```python
from build123d import *

# Parameters (mm, degrees)
SKETCH1_R           = 135.7
SKETCH1_R_2         = 4
BOSS_EXTRUDE1_DEPTH = 10.6
SKETCH3_R           = 4.3
SKETCH5_R           = 4.3


with BuildPart() as part:
    # Sketch1 → Boss-Extrude1 (new body)
    with BuildSketch(Plane(origin=(0, 0, 0), x_dir=(1, 0, 0), z_dir=(0, 1, 0))):
        with Locations(Location((0, 0, 0), (0, 0, 270))):
            Circle(SKETCH1_R)
        with Locations(Location((0, 0, 0), (0, 0, 270))):
            Circle(SKETCH1_R_2, mode=Mode.SUBTRACT)
        with BuildLine():
            Line((-9.028288874, 4.3), (-128.4, 4.3))
            ThreePointArc((-128.4, 4.3), (-111.259999551, 64.235990691), (-67.923909236, 109.047661846))
            Line((-67.923909236, 109.047661846), (-8.238053673, 5.668727518))
            ThreePointArc((-8.238053673, 5.668727518), (-8.660254038, 5), (-9.028288874, 4.3))
        make_face(mode=Mode.SUBTRACT)
        with BuildLine():
            Line((-9.028288874, -4.3), (-128.4, -4.3))
            ThreePointArc((-128.4, -4.3), (-111.259999551, -64.235990691), (-67.923909236, -109.047661846))
            Line((-67.923909236, -109.047661846), (-8.238053673, -5.668727518))
            ThreePointArc((-8.238053673, -5.668727518), (-8.660254038, -5), (-9.028288874, -4.3))
        make_face(mode=Mode.SUBTRACT)
        with BuildLine():
            Line((-0.790235201, 9.968727518), (-60.476090764, 113.347661846))
            ThreePointArc((-60.476090764, 113.347661846), (0, 128.471981381), (60.476090764, 113.347661846))
            Line((60.476090764, 113.347661846), (0.790235201, 9.968727518))
            ThreePointArc((0.790235201, 9.968727518), (0, 10), (-0.790235201, 9.968727518))
        make_face(mode=Mode.SUBTRACT)
        with BuildLine():
            Line((8.238053673, 5.668727518), (67.923909236, 109.047661846))
            ThreePointArc((67.923909236, 109.047661846), (111.259999551, 64.235990691), (128.4, 4.3))
            Line((128.4, 4.3), (9.028288874, 4.3))
            ThreePointArc((9.028288874, 4.3), (8.660254038, 5), (8.238053673, 5.668727518))
        make_face(mode=Mode.SUBTRACT)
        with BuildLine():
            Line((9.028288874, -4.3), (128.4, -4.3))
            ThreePointArc((128.4, -4.3), (111.259999551, -64.235990691), (67.923909236, -109.047661846))
            Line((67.923909236, -109.047661846), (8.238053673, -5.668727518))
            ThreePointArc((8.238053673, -5.668727518), (8.660254038, -5), (9.028288874, -4.3))
        make_face(mode=Mode.SUBTRACT)
        with BuildLine():
            Line((0.790235201, -9.968727518), (60.476090764, -113.347661846))
            ThreePointArc((60.476090764, -113.347661846), (0, -128.471981381), (-60.476090764, -113.347661846))
            Line((-60.476090764, -113.347661846), (-0.790235201, -9.968727518))
            ThreePointArc((-0.790235201, -9.968727518), (0, -10), (0.790235201, -9.968727518))
        make_face(mode=Mode.SUBTRACT)
    extrude(amount=BOSS_EXTRUDE1_DEPTH)

    # Sketch3 → Cut-Revolve1 (revolve, cut)
    with BuildSketch(Plane.XY, mode=Mode.PRIVATE) as cut_revolve1_sk:
        with Locations((135.7, 5.3)):
            Circle(SKETCH3_R)
    revolve(cut_revolve1_sk.sketch.rotate(Axis((0, 0, 0), (0, 1, 0)), 90), axis=Axis((0, 0, 0), (0, 1, 0)), mode=Mode.SUBTRACT)

    # Sketch5 → Revolve1 (revolve)
    with BuildSketch(Plane(origin=(0, 0, 0), x_dir=(0, 0, -1), z_dir=(1, 0, 0))):
        with Locations((135.7, 5.3)):
            Circle(SKETCH5_R)
    revolve(axis=Axis((0, 0, 0), (0, 1, 0)))


solid = part.part
```
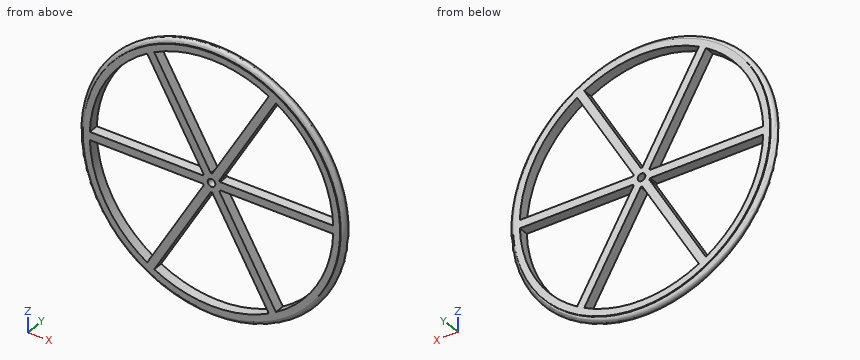
Could you check a few things on this model? Use its own coordinates, in mm. Give positions to 0.01 mm unless a question says otherwise; leave off trailing zeros. Order: outer loops, then holes, each group sorted by start corner. A loop starts at its lowest first (then second) coordinate and runs counter-clockwise, first axis right, second up.
Q1. I'm going to push flat-ended pins straight in: P1, Ø1, axis at x = 52.5, y = 4.5, coming from the +Z side; P2, Ø5.5, axis at x = -75, y = 6.5, coming from the +Z side; P3, Ø4, axis at x = -95, y = 9.5, coming from the -Z side. Where does each tip first touch, or does it pass through?
Q2. Suppose I cut it at C-C, the plane x = 122.5. Count the separate pieces of the cut face and the enclosed holes in it, and give its area (3 significant figures).
Q3. Suppose I cut it at B-B, the plane y = 3.5. Write out the boundary of the cut face in (x, z).
Q4. Suppose I cut it at A-A, the plane z = 0. Write out the boundary of the cut face in (x, y), and give its area (3 significant figures).
Q5. If I drill on line 1 along Z through (x, y) = (68, 6.75); line 2 along Z through (x, y) = (-45.5, 5); line 3 along Z through (x, y) = (21, 9.25), over which ranges is the centre line in solid material (lowest first)?
Solution:
1. P1: stops at z = 129.92
1. P2: stops at z = 119.83
1. P3: stops at z = -102.76
2. separate pieces: 3
2. enclosed holes: 0
2. area: 636 mm2
3. outline: circle Ø279.21 at (0, 0); hole (-128.4, -4.3) arc R128.47 ccw to (-67.92, -109.05) - (-8.24, -5.67) arc R10 cw to (-9.03, -4.3) - close; hole (-128.4, 4.3) - (-9.03, 4.3) arc R10 cw to (-8.24, 5.67) - (-67.92, 109.05) arc R128.47 ccw to start; hole (-60.48, -113.35) arc R128.47 ccw to (60.48, -113.35) - (0.79, -9.97) arc R10 cw to (-0.79, -9.97) - close; hole (-60.48, 113.35) - (-0.79, 9.97) arc R10 cw to (0.79, 9.97) - (60.48, 113.35) arc R128.47 ccw to start; hole circle Ø8 at (0, 0); hole (8.24, -5.67) - (67.92, -109.05) arc R128.47 ccw to (128.4, -4.3) - (9.03, -4.3) arc R10 cw to start; hole (8.24, 5.67) arc R10 cw to (9.03, 4.3) - (128.4, 4.3) arc R128.47 ccw to (67.92, 109.05) - close
4. outline: (-135.7, 0) - (-4, 0) - (-4, 10.6) - (-135.7, 10.6) - (-135.7, 9.6) arc R4.3 ccw to (-135.7, 1) - close; (4, 0) - (135.7, 0) - (135.7, 1) arc R4.3 ccw to (135.7, 9.6) - (135.7, 10.6) - (4, 10.6) - close
4. area: 2,850 mm2
5. line 1: z = -122.09 to -109, -4.3 to 4.3, 109 to 122.09
5. line 2: z = -132.39 to -120.14, -87.41 to -70.21, -4.3 to 4.3, 70.21 to 87.41, 120.14 to 132.39
5. line 3: z = -135.78 to -126.74, -44.97 to -27.77, -4.3 to 4.3, 27.77 to 44.97, 126.74 to 135.78
